Print and shaded views of the part. All mm, measured from the part's lowest x, y and z. A direction names the side the tool comes from. Coordinates: 2 decimals unless noted, no trailing zeros. Order: outer loops, then holes, each group sorted by start corner. A loop starts at its lowest first (then second) coordinate and runs counter-clockwise, first axis right, second up. Notation, with made-up numbers: M -39,65 L -12,65 A23 ccw -12,73 Z; hole C 87.25,-32.75 d1. An arc over 180 degrees is marked long. Return JSON: item names as keys, results as strings.
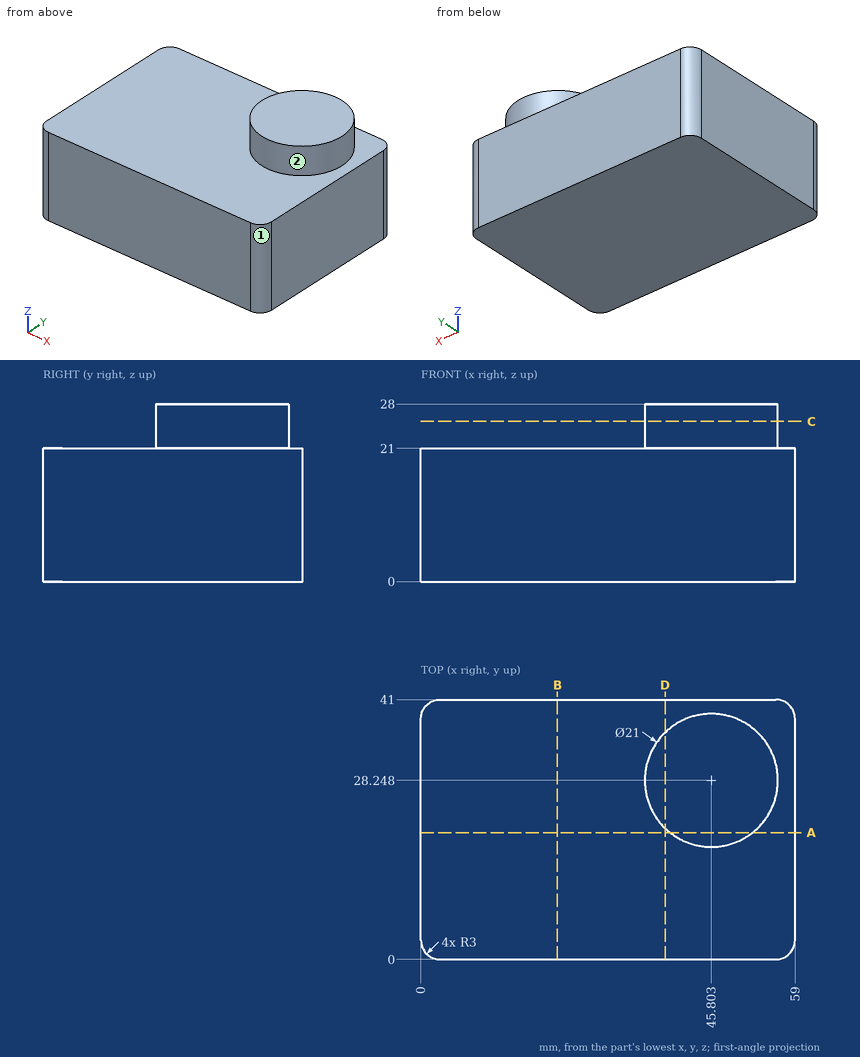
Item 1: Saw through at C-C (z = 25.25). Write the cut outline in (x, y).
Check result:
{"outline": "C 45.8,28.25 d21"}
Item 2: 3-axis set-ups, long thin cutter, end or side, ignore diameter. For the marked faces 1 and 2: which of +Z, -Z, +X, -X, +Y, -Y reach the whole face in a straight line?
Check result:
{"face 1": "+Z, -Z, +X, -Y", "face 2": "+Z"}
Item 3: Saw through at B-B (x = 21.5). Write the cut outline in (y, z).
Check result:
{"outline": "M 0,0 L 41,0 L 41,21 L 0,21 Z"}
Item 4: Wall check: line 1 (Z direction, x = 27, y = 20.5); line 2 (X direction, y = 27, z = 25.5); line 3 (X direction, y = 23.5, z = 22). Give the ranges that are in metal, low to high.
Check result:
{"line 1": "z = 0 to 21", "line 2": "x = 35.38 to 56.23", "line 3": "x = 36.44 to 55.17"}
Item 5: Saw through at D-D (x = 38.5). Write the cut outline in (y, z).
Check result:
{"outline": "M 0,0 L 41,0 L 41,21 L 35.79,21 L 35.79,28 L 20.7,28 L 20.7,21 L 0,21 Z"}
Item 6: Saw through at A-A (y = 20). Write the cut outline in (x, z) (1 decimal), and give its area (3 significant figures).
Check result:
{"outline": "M 0,0 L 59,0 L 59,21 L 52.3,21 L 52.3,28 L 39.3,28 L 39.3,21 L 0,21 Z", "area": "1,330 mm2"}
Item 7: Drop a flat-ended pin along its axis: pin 1 Ø3 at (x, y) = (49.5, 10.5) entering from +Z. Give the stop position or say it passes through.
Check result:
{"pin 1": "stops at z = 21"}
